Could you check a few things on this model? Use its own coordinates, in mm. Give positions to 0.01 mm unless a question says otherwise; leave off trailing zeros. Loops run counter-clockwise (first coordinate to the right, second up) from the corner with the lowest first, then second, coordinate; pieces in that order, holes last. Notation, with made-up numbers: (68.25, -18) -> (87.25, -18) arc R31 ccw to (87.25, 18) -> close; hole circle Ø5 at (3.25, -16.75). An arc over 180 degrees is marked (long way). Write each question's results on one line, items separated by ' | '. Start each with the question number.
Q1. If we section it at C-C, the plane x = 11: List the corners of the cut face in (y, z) for me, plus the area to 3 significant figures.
Q2. If we section it at A-A, the plane x = 6: List the corners of the cut face in (y, z) for me, plus the area to 3 significant figures.
Q3. Will these pins go through, and if not, where does the flat tip stop? P1, Ø5.5, axis at x = -1.5, y = -8, coming from the +Z side; P2, Ø0.5, axis at x = 5.5, z = 0.5, coming from the +Y side.
Q4. If we section it at B-B, the plane y = -8: List the corners of the cut face in (x, z) for me, plus the area to 3 significant figures.
Q5. If we section it at D-D, the plane y = -2: List the corners of the cut face in (x, z) for me.
Q6. If I drill on line 1 along Y through (x, z) = (8.5, 0.3); line 2 along X through (y, z) = (-8, 0.5); line 3 along Y through (x, z) = (11, 0.85), over which ranges is the centre line in solid material (lowest first)?
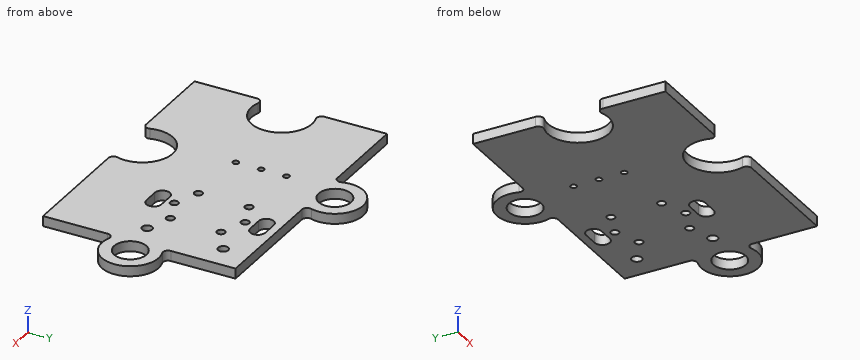
from build123d import *

# Parameters (mm, degrees)
CYLINDER012_R     = 0.5
CYLINDER012_DEPTH = 10
CYLINDER011_R     = 0.5
CYLINDER011_DEPTH = 10
CYLINDER010_R     = 0.3
CYLINDER010_DEPTH = 10
CYLINDER009_R     = 0.3
CYLINDER009_DEPTH = 10
CYLINDER008_R     = 0.3
CYLINDER008_DEPTH = 10
PAD004_DEPTH      = 5
PAD003_DEPTH      = 5
CYLINDER007_R     = 0.4
CYLINDER007_DEPTH = 10
CYLINDER006_R     = 0.4
CYLINDER006_DEPTH = 10
CYLINDER005_R     = 0.4
CYLINDER005_DEPTH = 10
CYLINDER004_R     = 0.4
CYLINDER004_DEPTH = 10
CYLINDER003_R     = 0.4
CYLINDER003_DEPTH = 10
CYLINDER002_R     = 0.4
CYLINDER002_DEPTH = 10
SKETCH_R          = 1.6
PAD_DEPTH         = 1
FILLET_R          = 0.5
FILLET001_R       = 0.5
FILLET002_R       = 0.5
FILLET003_R       = 0.5
FILLET004_R       = 0.5
FILLET005_R       = 0.5


with BuildPart() as cilindro012:
    # Cylinder012 → Cylinder012 (new body)
    with BuildSketch(Plane(origin=(11, -0.6, -2), x_dir=(1, 0, 0), z_dir=(0, 0, 1))):
        Circle(CYLINDER012_R)
    extrude(amount=CYLINDER012_DEPTH)


with BuildPart() as cilindro011:
    # Cylinder011 → Cylinder011 (new body)
    with BuildSketch(Plane(origin=(11, 6.9, -2), x_dir=(1, 0, 0), z_dir=(0, 0, 1))):
        Circle(CYLINDER011_R)
    extrude(amount=CYLINDER011_DEPTH)


with BuildPart() as cilindro010:
    # Cylinder010 → Cylinder010 (new body)
    with BuildSketch(Plane(origin=(-2.8, 0.5, -2), x_dir=(1, 0, 0), z_dir=(0, 0, 1))):
        Circle(CYLINDER010_R)
    extrude(amount=CYLINDER010_DEPTH)


with BuildPart() as cilindro009:
    # Cylinder009 → Cylinder009 (new body)
    with BuildSketch(Plane(origin=(-2.8, 3, -2), x_dir=(1, 0, 0), z_dir=(0, 0, 1))):
        Circle(CYLINDER009_R)
    extrude(amount=CYLINDER009_DEPTH)


with BuildPart() as cilindro008:
    # Cylinder008 → Cylinder008 (new body)
    with BuildSketch(Plane(origin=(-2.8, 5.5, -2), x_dir=(1, 0, 0), z_dir=(0, 0, 1))):
        Circle(CYLINDER008_R)
    extrude(amount=CYLINDER008_DEPTH)


with BuildPart() as pad004:
    # Sketch008 → Pad004 (new body)
    with BuildSketch(Plane(origin=(0, -9, 0), x_dir=(1, 0, 0), z_dir=(0, 0, 1))):
        with BuildLine():
            ThreePointArc((5.24484, 7.456211), (4.49484, 6.706211), (5.24484, 5.956211))
            Line((5.24484, 5.956211), (6.74484, 5.956211))
            ThreePointArc((6.74484, 5.956211), (7.49484, 6.706211), (6.74484, 7.456211))
            Line((5.24484, 7.456211), (6.74484, 7.456211))
        make_face()
    extrude(amount=PAD004_DEPTH)


with BuildPart() as pad003:
    # Sketch007 → Pad003 (new body)
    with BuildSketch(Plane(origin=(0, 1.25, 0), x_dir=(1, 0, 0), z_dir=(0, 0, 1))):
        with BuildLine():
            ThreePointArc((5.24484, 7.456211), (4.49484, 6.706211), (5.24484, 5.956211))
            Line((5.24484, 5.956211), (6.74484, 5.956211))
            ThreePointArc((6.74484, 5.956211), (7.49484, 6.706211), (6.74484, 7.456211))
            Line((5.24484, 7.456211), (6.74484, 7.456211))
        make_face()
    extrude(amount=PAD003_DEPTH)


with BuildPart() as cilindro007:
    # Cylinder007 → Cylinder007 (new body)
    with BuildSketch(Plane(origin=(6, 6.3, -2), x_dir=(1, 0, 0), z_dir=(0, 0, 1))):
        Circle(CYLINDER007_R)
    extrude(amount=CYLINDER007_DEPTH)


with BuildPart() as cilindro006:
    # Cylinder006 → Cylinder006 (new body)
    with BuildSketch(Plane(origin=(6, -0.7, -2), x_dir=(1, 0, 0), z_dir=(0, 0, 1))):
        Circle(CYLINDER006_R)
    extrude(amount=CYLINDER006_DEPTH)


with BuildPart() as cilindro005:
    # Cylinder005 → Cylinder005 (new body)
    with BuildSketch(Plane(origin=(8.5, 5.3, -2), x_dir=(1, 0, 0), z_dir=(0, 0, 1))):
        Circle(CYLINDER005_R)
    extrude(amount=CYLINDER005_DEPTH)


with BuildPart() as cilindro004:
    # Cylinder004 → Cylinder004 (new body)
    with BuildSketch(Plane(origin=(3.5, 5.3, -2), x_dir=(1, 0, 0), z_dir=(0, 0, 1))):
        Circle(CYLINDER004_R)
    extrude(amount=CYLINDER004_DEPTH)


with BuildPart() as cilindro003:
    # Cylinder003 → Cylinder003 (new body)
    with BuildSketch(Plane(origin=(8.5, 0.3, -2), x_dir=(1, 0, 0), z_dir=(0, 0, 1))):
        Circle(CYLINDER003_R)
    extrude(amount=CYLINDER003_DEPTH)


with BuildPart() as cilindro002:
    # Cylinder002 → Cylinder002 (new body)
    with BuildSketch(Plane(origin=(3.5, 0.3, -2), x_dir=(1, 0, 0), z_dir=(0, 0, 1))):
        Circle(CYLINDER002_R)
    extrude(amount=CYLINDER002_DEPTH)


with BuildPart() as baseled:
    # Sketch → Pad (new body)
    with BuildSketch(Plane.XY):
        with BuildLine():
            Line((-13.5, 9.5), (-3.864318, 9.5))
            ThreePointArc((0.864318, 9.5), (-1.5, 13.8), (-3.864318, 9.5))
            Line((0.864318, 9.5), (13.5, 9.5))
            Line((13.5, 9.5), (13.5, 2.297825))
            ThreePointArc((13.5, -2.297825), (17.9, 0), (13.5, 2.297825))
            Line((13.5, -2.297825), (13.5, -9.5))
            Line((13.5, -9.5), (1.098076, -9.5))
            ThreePointArc((1.098076, -9.5), (-1.5, -5), (-4.098076, -9.5))
            Line((-4.098076, -9.5), (-13.5, -9.5))
            Line((-13.5, -9.5), (-13.5, -2.537716))
            ThreePointArc((-13.5, -2.537716), (-8.9, 0), (-13.5, 2.537716))
            Line((-13.5, 2.537716), (-13.5, 9.5))
        make_face()
        with Locations((-1.5, 11)):
            Circle(SKETCH_R, mode=Mode.SUBTRACT)
        with Locations((15.1, 0)):
            Circle(SKETCH_R, mode=Mode.SUBTRACT)
    extrude(amount=PAD_DEPTH)

    # Fillet
    fillet_edges = [baseled.edges().sort_by_distance(p)[0] for p in [
        (-3.864318, 9.5, 0.5),
    ]]
    fillet(fillet_edges, radius=FILLET_R)

    # Fillet001
    fillet001_edges = [baseled.edges().sort_by_distance(p)[0] for p in [
        (0.864318, 9.5, 0.5),
    ]]
    fillet(fillet001_edges, radius=FILLET001_R)

    # Fillet002
    fillet002_edges = [baseled.edges().sort_by_distance(p)[0] for p in [
        (13.5, 2.297825, 0.5),
    ]]
    fillet(fillet002_edges, radius=FILLET002_R)

    # Fillet003
    fillet003_edges = [baseled.edges().sort_by_distance(p)[0] for p in [
        (13.5, -2.297825, 0.5),
    ]]
    fillet(fillet003_edges, radius=FILLET003_R)

    # Fillet004
    fillet004_edges = [baseled.edges().sort_by_distance(p)[0] for p in [
        (-4.098076, -9.5, 0.5),
    ]]
    fillet(fillet004_edges, radius=FILLET004_R)

    # Fillet005
    fillet005_edges = [baseled.edges().sort_by_distance(p)[0] for p in [
        (1.098076, -9.5, 0.5),
        (-13.5, -2.537716, 0.5),
        (-13.5, 2.537716, 0.5),
    ]]
    fillet(fillet005_edges, radius=FILLET005_R)

    # Cut003: cut Cilindro002
    add(cilindro002.part, mode=Mode.SUBTRACT)

    # Cut004: cut Cilindro003
    add(cilindro003.part, mode=Mode.SUBTRACT)

    # Cut005: cut Cilindro004
    add(cilindro004.part, mode=Mode.SUBTRACT)

    # Cut006: cut Cilindro005
    add(cilindro005.part, mode=Mode.SUBTRACT)

    # Cut007: cut Cilindro006
    add(cilindro006.part, mode=Mode.SUBTRACT)

    # Cut008: cut Cilindro007
    add(cilindro007.part, mode=Mode.SUBTRACT)

    # Cut009: cut Pad003
    add(pad003.part, mode=Mode.SUBTRACT)

    # Cut010: cut Pad004
    add(pad004.part, mode=Mode.SUBTRACT)

    # Cut011: cut Cilindro008
    add(cilindro008.part, mode=Mode.SUBTRACT)

    # Cut012: cut Cilindro009
    add(cilindro009.part, mode=Mode.SUBTRACT)

    # Cut013: cut Cilindro010
    add(cilindro010.part, mode=Mode.SUBTRACT)

    # Cut014: cut Cilindro011
    add(cilindro011.part, mode=Mode.SUBTRACT)

    # Cut015: cut Cilindro012
    add(cilindro012.part, mode=Mode.SUBTRACT)


solid = baseled.part
Final values:
1) outline: (-9.5, 0) -> (-1.1, 0) -> (-1.1, 1) -> (-9.5, 1) -> close; (-0.1, 0) -> (6.4, 0) -> (6.4, 1) -> (-0.1, 1) -> close; (7.4, 0) -> (9.5, 0) -> (9.5, 1) -> (7.4, 1) -> close | area: 17.0 mm²
2) outline: (-9.5, 0) -> (-3.04, 0) -> (-3.04, 1) -> (-9.5, 1) -> close; (-1.54, 0) -> (-1.1, 0) -> (-1.1, 1) -> (-1.54, 1) -> close; (-0.3, 0) -> (5.9, 0) -> (5.9, 1) -> (-0.3, 1) -> close; (6.7, 0) -> (7.21, 0) -> (7.21, 1) -> (6.7, 1) -> close; (8.71, 0) -> (9.5, 0) -> (9.5, 1) -> (8.71, 1) -> close | area: 14.4 mm²
3) P1: passes through | P2: stops at y = 9.5
4) outline: (-13.5, 0) -> (-4.5, 0) -> (-4.5, 1) -> (-13.5, 1) -> close; (1.5, 0) -> (13.5, 0) -> (13.5, 1) -> (1.5, 1) -> close | area: 21.0 mm²
5) outline: (-9.66, 0) -> (4.55, 0) -> (4.55, 1) -> (-9.66, 1) -> close; (7.43, 0) -> (17.06, 0) -> (17.06, 1) -> (7.43, 1) -> close
6) line 1: y = -9.5 to -0.1, 0.7 to 4.9, 5.7 to 9.5 | line 2: x = -13.5 to -4.5, 1.5 to 13.5 | line 3: y = -9.5 to -1.1, -0.1 to 6.4, 7.4 to 9.5
